For this review, use the dimensioned drawing (mm, ordinates from the lowest corner) and the shaded views. Round coordinates to 2 decimals unless told otherwise and drop trailing zeros. Order: outer loops, then holes, each group sorted by start corner. A loop starts at its lowest first (then second) coordinate and runs counter-clockwise, first axis right, second up. Notation, with made-up numbers: M 52.25,54.25 L 111.25,54.25 A26 ccw 111.25,90.25 Z; hole C 0.5,57.25 d11. An arc over 180 degrees is marked long. Use a Markdown table: item, result. Add a question column.
1. To check wall thickness, follow probe 1 along Y at (x, z) = (25, 4.35); probe 2 along Y at (x, z) = (47.5, 3.2); probe 3 along Y at (x, z) = (37.5, 0.3) (1 decimal). State the ranges of each line that lie inside material, in increasing order.
2. Consider section C-C on z = 3.35. Count the separate pieces of the cut face and the enclosed holes in it, then the cut area to 3 significant figures.
3. Consider section D-D on y = 14. State the section outline as (x, z) points.
4. Consider section A-A on x = 47.5. State the section outline as (y, z) points.
5. Consider section B-B on x = 70. State the section outline as (y, z) points.
6. Insertion check: P1, Ø2, axis at x = 7.5, y = 57.85, coming from the -Z side; P2, Ø5.5, axis at x = 7.5, y = 47.5, coming from the -Z side. Each pin has a flat end and moves straight along its axis. Give the tip position at first contact, or say it passes through.
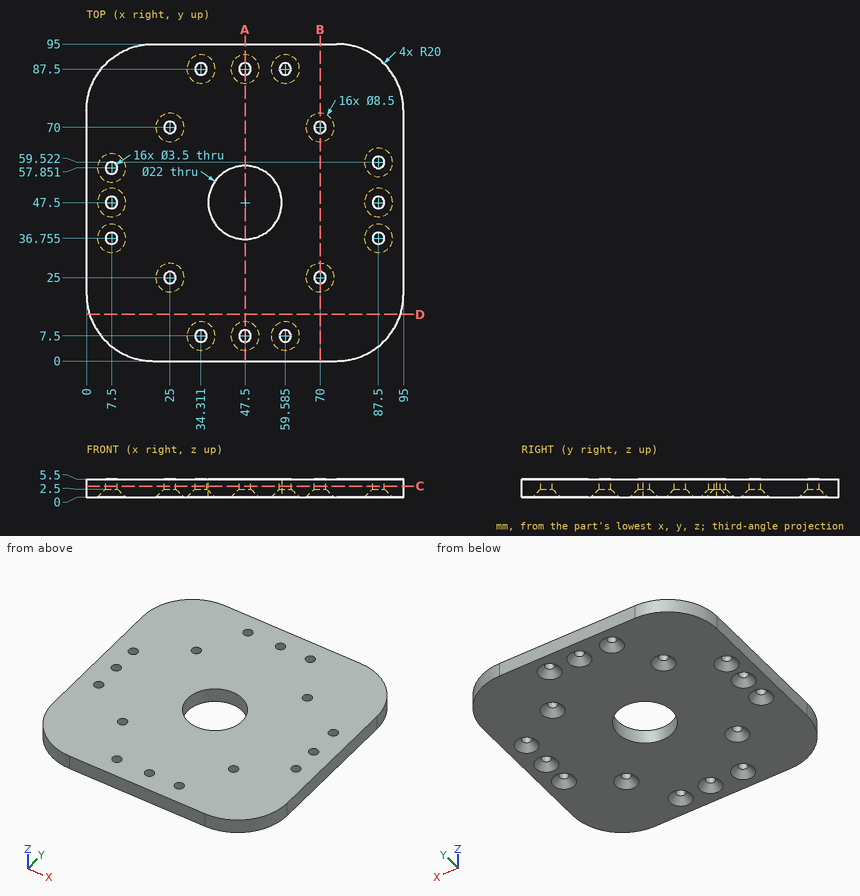
Answer block:
| question | item | result |
|---|---|---|
| 1 | probe 1 | 0 to 23.25, 26.75 to 68.25, 71.75 to 95 |
| 1 | probe 2 | 0 to 5.75, 9.25 to 36.5, 58.5 to 85.75, 89.25 to 95 |
| 1 | probe 3 | 0 to 5.2, 9.8 to 42.9, 52.1 to 85.2, 89.8 to 95 |
| 2 | separate pieces | 1 |
| 2 | enclosed holes | 17 |
| 2 | area | 8,150 mm^2 |
| 3 | outline | M 0.92,0 L 94.08,0 L 94.08,5.5 L 0.92,5.5 Z |
| 4 | outline | M 0,0 L 3.25,0 L 5.75,2.5 L 5.75,5.5 L 0,5.5 Z; M 9.25,2.5 L 11.75,0 L 36.5,0 L 36.5,5.5 L 9.25,5.5 Z; M 58.5,0 L 83.25,0 L 85.75,2.5 L 85.75,5.5 L 58.5,5.5 Z; M 89.25,2.5 L 91.75,0 L 95,0 L 95,5.5 L 89.25,5.5 Z |
| 5 | outline | M 0,0 L 20.75,0 L 23.25,2.5 L 23.25,5.5 L 0,5.5 Z; M 26.75,2.5 L 29.25,0 L 65.75,0 L 68.25,2.5 L 68.25,5.5 L 26.75,5.5 Z; M 71.75,2.5 L 74.25,0 L 95,0 L 95,5.5 L 71.75,5.5 Z |
| 6 | P1 | through |
| 6 | P2 | z = 1.5 |
